Build history of the part. All positions in model axes, mm. Face numbers are marked on the shaded views. A direction names the side the tool comes from. Give positions to 0.01 mm unless a question says otherwise; leave off trailing zeros. Order: outer loops, then holes, each group sorted by start corner. A loop starts at its lowest first (then second) coordinate and runs counter-clockwise, first axis right, second up. Notation, with made-up numbers: (88.5, -22) - (93.5, -22) arc R19 cw to (93.5, -9) - close; hole circle Ø9 at (-3, 67). An arc over 180 degrees is marked (long way). Answer in a Markdown table with one row per item.
```python
from build123d import *

# Parameters (mm, degrees)
SKETCH_1_R          = 6.05
EXTRUDE_1_DEPTH     = 4
SKETCH_2_R          = 7
EXTRUDE_2_DEPTH     = 0.5
SKETCH_3_R          = 6.05
EXTRUDE_3_DEPTH     = 4
SKETCH_5_R          = 5.5
EXTRUDE_4_DEPTH     = 0.5
SKETCH_6_R          = 5.05
EXTRUDE_5_DEPTH     = 4
CUT_EXTRUDE_1_DEPTH = 14


with BuildPart() as part:
    # 草图1 → 凸台-拉伸1 (new body)
    with BuildSketch(Plane.XY):
        with Locations((-0.75, 0)):
            Circle(SKETCH_1_R)
    extrude(amount=EXTRUDE_1_DEPTH)

    # 草图2 → 凸台-拉伸2 (add)
    with BuildSketch(Plane.XY.offset(4)):
        Circle(SKETCH_2_R)
    extrude(amount=EXTRUDE_2_DEPTH)

    # 草图3 → 凸台-拉伸3 (add)
    with BuildSketch(Plane.XY.offset(4.5)):
        with Locations((0.75, 0)):
            Circle(SKETCH_3_R)
    extrude(amount=EXTRUDE_3_DEPTH)

    # 草图5 → 凸台-拉伸4 (add)
    with BuildSketch(Plane(origin=(0, 0, 0), x_dir=(-1, 0, 0), z_dir=(0, 0, -1))):
        Circle(SKETCH_5_R)
    extrude(amount=EXTRUDE_4_DEPTH)

    # 草图6 → 凸台-拉伸5 (add)
    with BuildSketch(Plane(origin=(0, 0, -0.5), x_dir=(-1, 0, 0), z_dir=(0, 0, -1))):
        Circle(SKETCH_6_R)
    extrude(amount=EXTRUDE_5_DEPTH)

    # 草图4 → 切除-拉伸1 (cut, through all)
    with BuildSketch(Plane.XY.offset(8.5)):
        with BuildLine():
            ThreePointArc((4.05, 0), (-1.709856405, 3.671360929), (-2.606242506, -3.1))
            Line((-2.606242506, -3.1), (2.606242506, -3.1))
            ThreePointArc((2.606242506, -3.1), (3.671360929, -1.709856405), (4.05, 0))
        make_face()
    extrude(amount=-CUT_EXTRUDE_1_DEPTH, mode=Mode.SUBTRACT)


solid = part.part
```
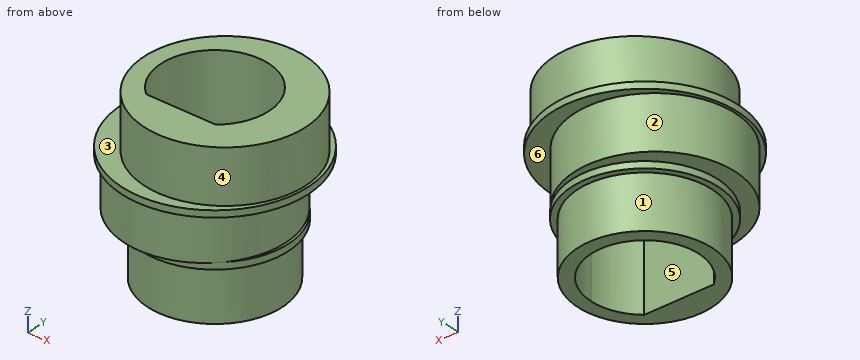
1. Which spindle directions (+Z, -Z, +X, -X, +Y, -Y) get a long thin tool onto all of the face, cutting with end or side? Do the marked faces 1, 2 and 3. Say none if no direction does.
Check result:
| item | result |
|---|---|
| face 1 | -Z |
| face 2 | none |
| face 3 | +Z |
2. Drop flat-ended pins along their axis: P1, Ø1, axis at y = 3, z = 2, coming from the +X side; P2, Ø1, axis at y = 4, z = 1, coming from the +X side. Give the stop position or say it passes through.
Check result:
| item | result |
|---|---|
| P1 | stops at x = 4.76 |
| P2 | stops at x = 4.18 |
3. Probe line 1 (X direction, y = 0, z = 0.5); line 2 (X direction, y = 0, z = -0.25); line 3 (Y direction, x = -2.25, z = -2.25). List the from-to ranges inside material, lowest first.
Check result:
| item | result |
|---|---|
| line 1 | x = -6.8 to -4.05, 4.05 to 5.3 |
| line 2 | x = -5.5 to -4.05, 4.05 to 5.5 |
| line 3 | y = -4.52 to -3.1, 3.37 to 4.52 |
4. Cut at A-A on x = 0. Write the cut outline in (y, z).
Check result:
| item | result |
|---|---|
| outline | (-7, 4) - (-6, 4) - (-6, 0) - (-5.5, 0) - (-5.5, -0.5) - (-5.05, -0.5) - (-5.05, -4.5) - (-3.1, -4.5) - (-3.1, 8.5) - (-6, 8.5) - (-6, 4.5) - (-7, 4.5) - close; (4.05, -4.5) - (5.05, -4.5) - (5.05, -0.5) - (5.5, -0.5) - (5.5, 0) - (6, 0) - (6, 4) - (7, 4) - (7, 4.5) - (6, 4.5) - (6, 8.5) - (4.05, 8.5) - close |
5. Cut at D-D on x = -4.25. Write the cut outline in (y, z), and give its area (3 significant figures).
Check result:
| item | result |
|---|---|
| outline | (-5.56, 4) - (-4.93, 4) - (-4.93, 0) - (-3.49, 0) - (-3.49, -0.5) - (-2.73, -0.5) - (-2.73, -4.5) - (2.73, -4.5) - (2.73, -0.5) - (3.49, -0.5) - (3.49, 0) - (4.93, 0) - (4.93, 4) - (5.56, 4) - (5.56, 4.5) - (3.41, 4.5) - (3.41, 8.5) - (-3.41, 8.5) - (-3.41, 4.5) - (-5.56, 4.5) - close |
| area | 97.6 mm² |
6. Cut at B-B on y = 1.5. Write the cut outline in (x, z).
Check result:
| item | result |
|---|---|
| outline | (-6.84, 4) - (-6.61, 4) - (-6.61, 0) - (-5.29, 0) - (-5.29, -0.5) - (-4.82, -0.5) - (-4.82, -4.5) - (-3.76, -4.5) - (-3.76, 8.5) - (-5.11, 8.5) - (-5.11, 4.5) - (-6.84, 4.5) - close; (3.76, -4.5) - (4.82, -4.5) - (4.82, -0.5) - (5.29, -0.5) - (5.29, 0) - (5.11, 0) - (5.11, 4) - (6.84, 4) - (6.84, 4.5) - (6.61, 4.5) - (6.61, 8.5) - (3.76, 8.5) - close |
7. Cut at C-C on z = 3.25. Write the cut outline in (x, y).
Check result:
| item | result |
|---|---|
| outline | circle Ø12.1 at (-0.75, 0); hole (-2.61, -3.1) - (2.61, -3.1) arc R4.05 ccw (long way) to start |
8. Two-plate mould, pull along X, no slides. Class the marked faces 4, 5 and 6: +X half, -X half, draft (parallel to the pull), parting line (faces both ways), or undercut.
Check result:
| item | result |
|---|---|
| face 4 | parting line |
| face 5 | undercut |
| face 6 | draft |
